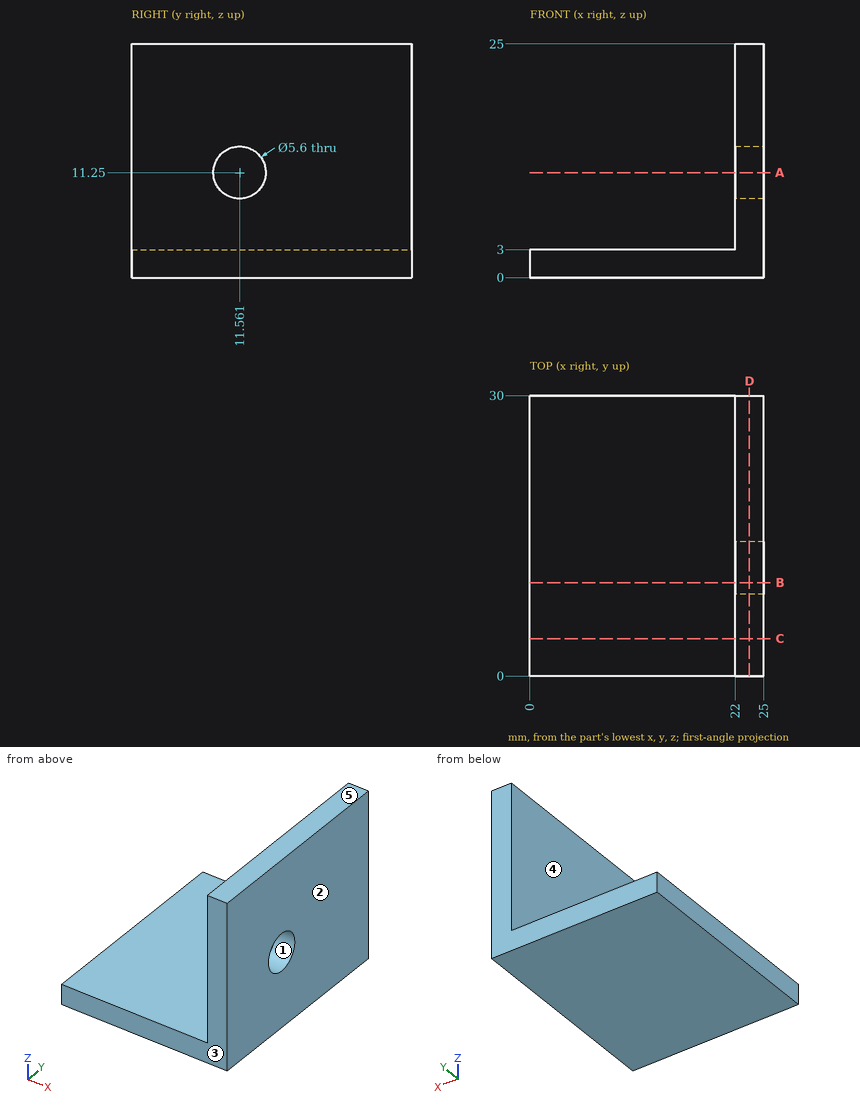
Design review of the part shown in the three views and the two pictorial views. Dimensions are in mm from the part's minimum x, y and z. A direction names the side the tool comes from. Coordinates: 2 decimals unless noted, no trailing zeros. Loops run counter-clockwise (first coordinate to the right, second up) from the corner with the lowest first, then second, coordinate; pieces in that order, holes last. Notation, with made-up numbers: (31, 26.5) - (80, 26.5) arc R12 ccw to (80, 46.5) - close; hole circle Ø5 at (-1, -14). An arc over 180 degrees is marked (long way). Use a Markdown table: item, result. Add a question column.
Item 1: We need section B-B (y = 10). Give the boundary of the cut face in (x, z).
Item 2: For line 1 (Z direction, x = 16.25, y = 2.5); line 2 (X direction, y = 14.5, z = 8), list the stretches that pass through material, from the lowest coordinate up.
Item 3: We need section C-C (y = 4). Give the boundary of the cut face in (x, z).
Item 4: Tool access review of the marked faces 4 and 5: name each direction out of +Z, -Z, +X, -X, +Y, -Y from which nothing blocks a thin tool from reaching the whole face with its end or side.
Item 5: Mouldability with a two-part tool opening along Y and no side actions: class the marked faces 1, 2 and 3 as pulls with the +Y half, pulls with the -Y half, needs draft (parallel to the pull), parting line crosses it, or undercut.
Item 6: We need section D-D (x = 23.5). Give the boundary of the cut face in (y, z).
Item 7: Insertion check: pin 1 Ø4 at (x, y) = (9, 13) entering from +Z; pin 2 Ø7.5 at (y, z) = (11.56, 11.25) entering from -X; pin 3 Ø8 at (x, y) = (7.5, 8) entering from -Z. Each pin has a flat end and moves straight along its axis. Give the tip position at first contact, or say it passes through.
Item 8: We need section A-A (z = 11.25). Give the boundary of the cut face in (x, y).
Results list:
| question | item | result |
|---|---|---|
| 1 | outline | (0, 0) - (25, 0) - (25, 8.93) - (22, 8.93) - (22, 3) - (0, 3) - close; (22, 13.57) - (25, 13.57) - (25, 25) - (22, 25) - close |
| 2 | line 1 | z = 0 to 3 |
| 2 | line 2 | x = 22 to 25 |
| 3 | outline | (0, 0) - (25, 0) - (25, 25) - (22, 25) - (22, 3) - (0, 3) - close |
| 4 | face 4 | +Z, -X, +Y, -Y |
| 4 | face 5 | +Z, +X, -X, +Y, -Y |
| 5 | face 1 | undercut |
| 5 | face 2 | needs draft |
| 5 | face 3 | pulls with the -Y half |
| 6 | outline | (0, 0) - (30, 0) - (30, 25) - (0, 25) - close; hole circle Ø5.6 at (11.56, 11.25) |
| 7 | pin 1 | stops at z = 3 |
| 7 | pin 2 | stops at x = 22 |
| 7 | pin 3 | stops at z = 0 |
| 8 | outline | (22, 0) - (25, 0) - (25, 8.76) - (22, 8.76) - close; (22, 14.36) - (25, 14.36) - (25, 30) - (22, 30) - close |
